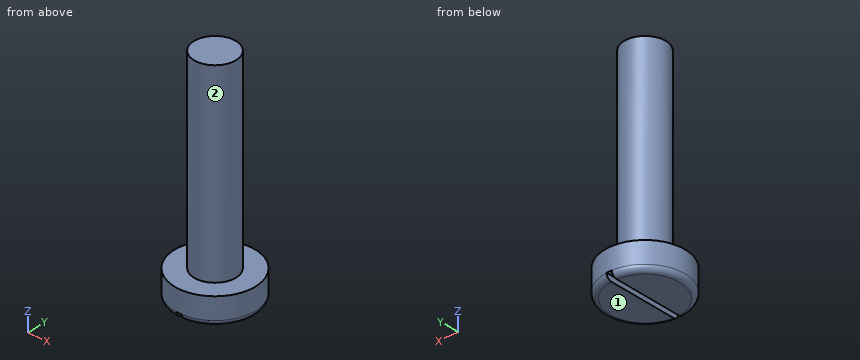
from build123d import *

# Parameters (mm, degrees)
CUT_EXTRUDE1_DEPTH = 0.254
FILLET1_R          = 0.254


with BuildPart() as part:
    # Sketch3 → Revolve1 (revolve)
    with BuildSketch(Plane(origin=(0, 0, 0), x_dir=(0, 0, -1), z_dir=(1, 0, 0)), mode=Mode.PRIVATE) as revolve1_sk:
        Polygon((0, 1.905), (1.27, 1.905), (1.27, 0), (0, 0), (-9.0932, 0), (-9.0932, 0.9906), (0, 0.9906), align=None)
    revolve(revolve1_sk.sketch.rotate(Axis((0, 0, 55), (0, 0, -1)), 90), axis=Axis((0, 0, 55), (0, 0, -1)))

    # Sketch4 → Cut-Extrude1 (cut)
    with BuildSketch(Plane(origin=(0, 0, -1.27), x_dir=(-1, 0, 0), z_dir=(0, 0, -1))):
        with BuildLine():
            Line((0, -1.905), (0, 1.905))
            ThreePointArc((0, 1.905), (-0.063535, 1.90394), (-0.127, 1.900762))
            Line((-0.127, 1.900762), (-0.127, -1.900762))
            ThreePointArc((-0.127, -1.900762), (-0.063535, -1.90394), (0, -1.905))
        make_face()
        with BuildLine():
            ThreePointArc((0.127, 1.900762), (0.063535, 1.90394), (0, 1.905))
            Line((0, 1.905), (0, -1.905))
            ThreePointArc((0, -1.905), (0.063535, -1.90394), (0.127, -1.900762))
            Line((0.127, -1.900762), (0.127, 1.900762))
        make_face()
    extrude(amount=-CUT_EXTRUDE1_DEPTH, mode=Mode.SUBTRACT)

    # Fillet1
    fillet1_edges = [part.edges().sort_by_distance(p)[0] for p in [
        (-1.905, 0, -1.27),
        (1.391215, 1.301363, -1.27),
    ]]
    fillet(fillet1_edges, radius=FILLET1_R)


solid = part.part
Geometry check sheet. Reference: the model listing, model coordinates, mm. Face numbers are marked on the shaded views. A direction names the side the tool comes from. Round coordinates to 2 decimals unless told otherwise and drop trailing zeros. Order: outer loops, then holes, each group sorted by start corner. A loop starts at its lowest first (then second) coordinate and runs counter-clockwise, first axis right, second up. Notation, with made-up numbers: M 4.25,58.25 L 49.25,58.25 A20 ccw 49.25,93.25 Z; hole C -19,16.25 d6. An arc over 180 degrees is marked long. Answer in a Markdown table with one row per item.
(1) Sectioned sample at C-C, the plane z = 5.25. Record the cut outline in (x, y), and give its area (3 significant figures).
Responses:
| item | result |
|---|---|
| outline | C 0,0 d1.98 |
| area | 3.08 mm² |
(2) Sectioned sample at A-A, the plane x = 0. Record the cut outline in (y, z) (3 decimals), and give its area (3 significant figures).
Responses:
| item | result |
|---|---|
| outline | M -1.905,-1.016 L 1.905,-1.016 L 1.905,0 L 0.991,0 L 0.991,9.093 L -0.991,9.093 L -0.991,0 L -1.905,0 Z |
| area | 21.9 mm² |
(3) Scan lines: probe 1 along Z at (x, y) = (1.4, 0.55); probe 2 along Z at (x, y) = (0, 0.5); probe 3 along X at (y, z) = (0.05, 0.75). Record each from-to range of solid material in increasing order. Write a range as from..to.
Responses:
| item | result |
|---|---|
| probe 1 | z = -1.27..0 |
| probe 2 | z = -1.02..9.09 |
| probe 3 | x = -0.99..0.99 |
(4) Sectioned sample at B-B, the plane y = 0. Record the cut outline in (x, z) (3 decimals), and give its area (3 significant figures).
Responses:
| item | result |
|---|---|
| outline | M -1.905,-1.016 A0.254 ccw -1.651,-1.27 L -0.127,-1.27 L -0.127,-1.016 L 0.127,-1.016 L 0.127,-1.27 L 1.651,-1.27 A0.254 ccw 1.905,-1.016 L 1.905,0 L 0.991,0 L 0.991,9.093 L -0.991,9.093 L -0.991,0 L -1.905,0 Z |
| area | 22.8 mm² |
(5) Tool access check on the marked faces 1 and 2. Record the directions out of +Z, -Z, +X, -X, +Y, -Y that give a thin tool (end or side, any length) a straight path to the whole face; none if there is none.
Responses:
| item | result |
|---|---|
| face 1 | -Z, +X, -X, +Y, -Y |
| face 2 | +Z |
